from build123d import *

# Parameters (mm, degrees)
F0_W     = 26.2
F0_H     = 25.2
F1_DEPTH = 98
F2_T     = -2
F3_R     = 9
F4_DEPTH = 2
F7_DEPTH = 2
F8_R     = 5


with BuildPart() as f1:
    # F0 (on Top) → F1 (new body)
    with BuildSketch(Plane.XY):
        Rectangle(F0_W, F0_H)
    extrude(amount=-F1_DEPTH)

    # F2
    f2_openings = [f1.faces().sort_by_distance(p)[0] for p in [
        (0, 0, 0),
    ]]
    offset(amount=F2_T, openings=f2_openings)

    # F3 (on face) → F4 (cut)
    with BuildSketch(Plane(origin=(0, 0, -98), x_dir=(1, 0, 0), z_dir=(0, 0, -1))):
        Circle(F3_R)
    extrude(amount=-F4_DEPTH, mode=Mode.SUBTRACT)

    # F6 (on face) → F7 (cut)
    with BuildSketch(Plane.XZ.offset(12.6)):
        Polygon((-8, -26.982739), (8, -26.982739), (8, -5.982739), (0, -5.982739), (-8, -5.982739), align=None)
    extrude(amount=-F7_DEPTH, mode=Mode.SUBTRACT)

    # F8
    f8_edges = [f1.edges().sort_by_distance(p)[0] for p in [
        (13.1, -12.6, -49),
        (-13.1, -12.6, -49),
        (-13.1, 12.6, -49),
        (13.1, 12.6, -49),
    ]]
    fillet(f8_edges, radius=F8_R)


solid = f1.part
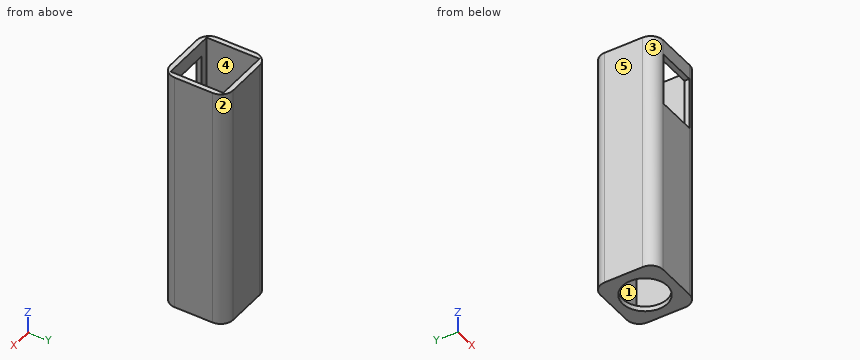
Read the model definition and answer for the solid it produces. Units are mm, in the model's axes. Face numbers are marked on the shaded views. A direction names the side the tool comes from. Give positions to 0.01 mm unless a question says otherwise; leave off trailing zeros. Write each loop counter-clockwise with the first axis right and the second up, starting at its lowest first coordinate (ties: lowest second). Pieces come first, ordered by that corner, then holes. Notation, with made-up numbers: (68.25, -35) - (77.25, -35) arc R28 cw to (77.25, -9) - close; hole circle Ø7 at (67, -3). An arc over 180 degrees is marked (long way). Use CSV: the item, a comma, the result in double quotes. Start each with the question number.
(1) Find section A-A (x = 0). Give the vertices of the cut face in (y, z), plus the area to 3 significant figures.
(2) Determine the mould class of the marked faces 3, 4 and 5 for opening direction Y: +Y half, -Y half, draft (parallel to the pull), parting line (faces both ways), or undercut.
(3) Find section B-B (y = 0). Give the vertices of the cut face in (x, z), plus the area to 3 significant figures.
(4) Find section C-C (z = -91.5). Give the vertices of the cut face in (x, y), plus the area to 3 significant figures.
(5) Given P1, Ø1.6, axis at y = -11.5, z = -14, coming from the -X side; P2, Ø3, axis at y = 9.5, z = -64, coming from the -X side; P3, Ø2, axis at y = -12, z = -13, coming from the +X side, each flat-ended and moving along its own axis, determine where each tip first touches the part or whether it passes through.
(6) Consider line 1 along X through (y, z) = (0, -96.65); line 2 along Y through (x, z) = (0, -97); line 3 along X through (y, z) = (-6.5, -78.5). Determine where each line is inside the solid, lowest interval first.
(7) Find section D-D (z = -25). Give the vertices of the cut face in (x, y), plus the area to 3 significant figures.
(8) For the marked faces 1 and 2, determine the directions among +Z, -Z, +X, -X, +Y, -Y from which every point of the face is accessible in a straight line to the end or side of a thin tool.
Findings below:
1,outline,"(-12.6, -98) - (-9, -98) - (-9, -96) - (-10.6, -96) - (-10.6, -26.98) - (-12.6, -26.98) - close; (-12.6, -5.98) - (-10.6, -5.98) - (-10.6, 0) - (-12.6, 0) - close; (9, -98) - (12.6, -98) - (12.6, 0) - (10.6, 0) - (10.6, -96) - (9, -96) - close"
1,area,"356 mm2"
2,face 3,"-Y half"
2,face 4,"undercut"
2,face 5,"draft"
3,outline,"(-13.1, -98) - (-9, -98) - (-9, -96) - (-11.1, -96) - (-11.1, 0) - (-13.1, 0) - close; (9, -98) - (13.1, -98) - (13.1, 0) - (11.1, 0) - (11.1, -96) - (9, -96) - close"
3,area,"400 mm2"
4,outline,"(-13.1, -7.6) arc R5 ccw to (-8.1, -12.6) - (8.1, -12.6) arc R5 ccw to (13.1, -7.6) - (13.1, 7.6) arc R5 ccw to (8.1, 12.6) - (-8.1, 12.6) arc R5 ccw to (-13.1, 7.6) - close; hole (-11.1, -10.6) - (11.1, -10.6) - (11.1, 10.6) - (-11.1, 10.6) - close"
4,area,"168 mm2"
5,P1,"x = -12.02"
5,P2,"x = -13.08"
5,P3,"x = 11.77"
6,line 1,"-13.1 to -9, 9 to 13.1"
6,line 2,"-12.6 to -9, 9 to 12.6"
6,line 3,"-13.1 to -11.1, 11.1 to 13.1"
7,outline,"(-13.1, -7.6) arc R5 ccw to (-8.1, -12.6) - (-8, -12.6) - (-8, -10.6) - (-11.1, -10.6) - (-11.1, 10.6) - (11.1, 10.6) - (11.1, -10.6) - (8, -10.6) - (8, -12.6) - (8.1, -12.6) arc R5 ccw to (13.1, -7.6) - (13.1, 7.6) arc R5 ccw to (8.1, 12.6) - (-8.1, 12.6) arc R5 ccw to (-13.1, 7.6) - close"
7,area,"136 mm2"
8,face 1,"+Z"
8,face 2,"+Z, -Z, +X, +Y"
